Design review of the part built by this model. Coordinates are the model's own, in mm. A direction names the side the tool comes from. Coordinates: 2 decimals unless noted, no trailing zeros. Write each loop counter-clockwise with the first axis right and the second up, starting at its lowest first coordinate (ties: lowest second). Pieces come first, ordered by that corner, then holes. Notation, with made-up numbers: (51.5, 29) - (56.5, 29) arc R20 ccw to (56.5, 50) - close; hole circle Ø11 at (66, 55.25). An arc over 180 degrees is marked (long way). Answer as CSV lines item,"result". Start each with the question number.
Q1. We need section D-D (x = 29). Write out the cut boundary in (y, z), plus the area to 3 significant figures.
Q2. Clearance check with flat-ended pins moving along their axes: pin 1 (10 mm diameter, centred on x = 23, y = 8, fed in from +Z); pin 2 (0.9 mm diameter, centred on x = 18, z = 7, fed in from +Y); pin 3 (4.5 mm diameter, centred on x = 25, y = 20, fed in from +Z). State where each tip first meets the part, or that it passes through.
Q3. For line 1 along Y through (x, z) = (22, 6.8); line 2 along X through (y, z) = (7.5, 0.35); line 3 along Y through (x, z) = (22, 0.3), list the stretches that pass through material, from the lowest coordinate up. Write a range as [from, to].
Q4. Mouldability with a two-part tool opening along Y and no side actions: class faces 1 (the face through (20.002, 7.412, 5.634)), 2 (the face through (20.328, 6.218, 3.093)), 3 (the face through (22, 23, 5)), 4 (the face through (22, 30, 2)) as pulls with the +Y half, pulls with the -Y half, needs draft (parallel to the pull), parting line crosses it, or undercut.
Q5. We need section C-C (z = 6.75). Write out the cut boundary in (x, y), plus the area to 3 significant figures.
Q6. Machinability: for faces 5 (the face through (22, 15, 6)), 6 (the face through (21.08, 11.65, 0.51)), 7 (the face through (0, 15, 3)), which of the approach directions +Z, -Z, +X, -X, +Y, -Y give a long, thin tool a straight path to every point of the face, cutting with its end or side? Answer none if there is none.
Q7. We need section B-B (y = 7.5). Write out the cut boundary in (x, z), plus the area to 3 significant figures.
Q8. We need section A-A (x = 22). Write out the cut boundary in (y, z).
from build123d import *

# Parameters (mm, degrees)
CYLINDER007_R             = 4.25
CYLINDER007_DEPTH         = 10
CYLINDER008_R             = 2
CYLINDER008_DEPTH         = 10
FUSION008_PLACEMENT_ANGLE = 180
CYLINDER009_R             = 4.25
CYLINDER009_DEPTH         = 8
CYLINDER001_R             = 4.25
CYLINDER001_DEPTH         = 10
CYLINDER_R                = 2
CYLINDER_DEPTH            = 10
BOX001_W                  = 44
BOX001_H                  = 15
BOX001_DEPTH              = 8
BOX_W                     = 44
BOX_H                     = 30
BOX_DEPTH                 = 5
CHAMFER_SIZE              = 2.2
CHAMFER003_SIZE           = 2.2


with BuildPart() as cylinder007:
    # Cylinder007 → Cylinder007 (new body)
    with BuildSketch(Plane(origin=(22, 7.5, 7), x_dir=(1, 0, 0), z_dir=(0, 0, 1))):
        Circle(CYLINDER007_R)
    extrude(amount=CYLINDER007_DEPTH)


with BuildPart() as fusion008:
    # Cylinder008 → Cylinder008 (new body)
    with BuildSketch(Plane(origin=(22, 7.5, 0), x_dir=(1, 0, 0), z_dir=(0, 0, 1))):
        Circle(CYLINDER008_R)
    extrude(amount=CYLINDER008_DEPTH)

    # Fusion008: union Cylinder007
    add(cylinder007.part)


with BuildPart() as fusion008_1:
    # Fusion008 placement: moved
    add(fusion008.part.moved(Location((0, 15, 8))).rotate(Axis((0, 15, 8), (1, 0, 0)), FUSION008_PLACEMENT_ANGLE))


with BuildPart() as cylinder009:
    # Cylinder009 → Cylinder009 (new body)
    with BuildSketch(Plane(origin=(22, 7.5, 0), x_dir=(1, 0, 0), z_dir=(0, 0, 1))):
        Circle(CYLINDER009_R)
    extrude(amount=CYLINDER009_DEPTH)


with BuildPart() as cylinder001:
    # Cylinder001 → Cylinder001 (new body)
    with BuildSketch(Plane(origin=(22, 7.5, 7), x_dir=(1, 0, 0), z_dir=(0, 0, 1))):
        Circle(CYLINDER001_R)
    extrude(amount=CYLINDER001_DEPTH)


with BuildPart() as fusion001:
    # Cylinder → Cylinder (new body)
    with BuildSketch(Plane(origin=(22, 7.5, 0), x_dir=(1, 0, 0), z_dir=(0, 0, 1))):
        Circle(CYLINDER_R)
    extrude(amount=CYLINDER_DEPTH)

    # Fusion001: union Cylinder001
    add(cylinder001.part)


with BuildPart() as cube001:
    # Box001 → Box001 (new body)
    with BuildSketch(Plane.XY):
        with Locations((22, 7.5)):
            Rectangle(BOX001_W, BOX001_H)
    extrude(amount=BOX001_DEPTH)


with BuildPart() as chamfer003:
    # Box → Box (new body)
    with BuildSketch(Plane.XY):
        with Locations((22, 15)):
            Rectangle(BOX_W, BOX_H)
    extrude(amount=BOX_DEPTH)

    # Fusion: union Cube001
    add(cube001.part)

    # Cut: cut Fusion001
    add(fusion001.part, mode=Mode.SUBTRACT)

    # Chamfer
    chamfer_edges = [chamfer003.edges().sort_by_distance(p)[0] for p in [
        (20, 7.5, 7),
    ]]
    chamfer(chamfer_edges, length=CHAMFER_SIZE)

    # Fusion009: union Cylinder009
    add(cylinder009.part)

    # Cut003: cut Fusion008
    add(fusion008_1.part, mode=Mode.SUBTRACT)

    # Chamfer003
    chamfer003_edges = [chamfer003.edges().sort_by_distance(p)[0] for p in [
        (20, 7.5, 1),
    ]]
    chamfer(chamfer003_edges, length=CHAMFER003_SIZE)


solid = chamfer003.part
Results list:
1,outline,"(0, 0) - (30, 0) - (30, 5) - (15, 5) - (15, 8) - (0, 8) - close"
1,area,"195 mm2"
2,pin 1,"stops at z = 8"
2,pin 2,"stops at y = 15"
2,pin 3,"stops at z = 5"
3,line 1,"y = [0, 5.5], [9.5, 15]"
3,line 2,"x = [0, 17.75], [26.25, 44]"
3,line 3,"y = [0, 3.25], [11.75, 30]"
4,face 1,"undercut"
4,face 2,"undercut"
4,face 3,"needs draft"
4,face 4,"pulls with the +Y half"
5,outline,"(0, 0) - (44, 0) - (44, 15) - (0, 15) - close; hole circle Ø4 at (22, 7.5)"
5,area,"647 mm2"
6,face 5,"+Z, +X, -X, +Y"
6,face 6,"-Z"
6,face 7,"+Z, -Z, -X, +Y, -Y"
7,outline,"(0, 0) - (17.75, 0) - (17.75, 1) - (17.8, 1) - (20, 3.2) - (20, 8) - (0, 8) - close; (24, 3.2) - (26.2, 1) - (26.25, 1) - (26.25, 0) - (44, 0) - (44, 8) - (24, 8) - close"
7,area,"311 mm2"
8,outline,"(0, 0) - (3.25, 0) - (3.25, 1) - (3.3, 1) - (5.5, 3.2) - (5.5, 8) - (0, 8) - close; (9.5, 3.2) - (11.7, 1) - (11.75, 1) - (11.75, 0) - (30, 0) - (30, 5) - (15, 5) - (15, 8) - (9.5, 8) - close"
